Can you work these out from the model? Positions are in its coordinate system, mm. Coordinates: 2 decimals unless noted, no trailing zeros. Order: outer loops, then holes, each group sorted by start corner. A loop starts at its lowest first (then second) coordinate and runs counter-clockwise, first axis right, second up. Notation, with made-up numbers: (-15, 28.5) -> (40, 28.5) arc R24 cw to (40, 67.5) -> close; hole circle Ø2 at (73, 11.5). An arc over 180 degrees is marked (long way). Use a Markdown table: item, result. Add a question column.
1. Suppose I cut it at C-C, the plane z = 5.35. List the corners of the cut face in (x, y) for me, then the cut area to 3 significant figures.
2. Suppose I cut it at B-B, the plane x = -12.5. List the corners of the cut face in (y, z) for me, then the cut area to 3 significant figures.
3. Suppose I cut it at D-D, the plane z = 2.5. List the corners of the cut face in (x, y) for me, then the cut area to 3 significant figures.
4. We'd pull the mould along Y, two halves only. Please class faces 1 (the flat face through (-26, 41, 6.4)), 2 (the cylindrical face through (12.776, 26.96, 3.358)), 3 (the cylindrical face through (-17.594, -3.941, 2.372)): pulls with the +Y half, pulls with the -Y half, needs draft (parallel to the pull), parting line crosses it, or undercut.
5. Suppose I cut it at A-A, the plane y = 19. List the corners of the cut face in (x, z) for me, then the cut area to 3 significant figures.
6. If I drill on line 1 along Y through (x, z) = (-12.5, 1.7); line 2 along Y through (x, z) = (-21, 1.55); line 3 along X through (y, z) = (8, 0.7), over which ranges is the centre line in solid material (lowest first)? Write a range as from..to.
7. For pin 1 Ø1 at (x, z) = (2, 3.5) entering from -Y, with a flat end and sliding along its axis, tell me the tip position at first contact or that it passes through.
```python
from build123d import *

# Parameters (mm, degrees)
CYLINDER025_R     = 23.5
CYLINDER025_DEPTH = 6
CYLINDER024_R     = 26.5
CYLINDER024_DEPTH = 6
CHAMFER013_SIZE   = 2


with BuildPart() as obj1:
    # Cylinder025 → Cylinder025 (new body)
    with BuildSketch(Plane(origin=(-12.5, 19, -10.6), x_dir=(1, 0, 0), z_dir=(0, 0, 1))):
        Circle(CYLINDER025_R)
    extrude(amount=CYLINDER025_DEPTH)


with BuildPart() as obj2:
    # Cylinder024 → Cylinder024 (new body)
    with BuildSketch(Plane(origin=(-12.5, 19, -10.6), x_dir=(1, 0, 0), z_dir=(0, 0, 1))):
        Circle(CYLINDER024_R)
    extrude(amount=CYLINDER024_DEPTH)

    # Cut012: cut obj1
    add(obj1.part, mode=Mode.SUBTRACT)


with BuildPart() as obj2_1:
    # Cut012 placement: moved
    add(obj2.part.moved(Location((0, 0, 11))))

    # Chamfer013
    chamfer013_edges = [obj2_1.edges().sort_by_distance(p)[0] for p in [
        (-36, 19, 6.4),
    ]]
    chamfer(chamfer013_edges, length=CHAMFER013_SIZE)


solid = obj2_1.part
```
Worked out:
| question | item | result |
|---|---|---|
| 1 | outline | circle Ø53 at (-12.5, 19); hole circle Ø48.9 at (-12.5, 19) |
| 1 | area | 328 mm² |
| 2 | outline | (-7.5, 0.4) -> (-4.5, 0.4) -> (-4.5, 4.4) -> (-6.5, 6.4) -> (-7.5, 6.4) -> close; (42.5, 0.4) -> (45.5, 0.4) -> (45.5, 6.4) -> (44.5, 6.4) -> (42.5, 4.4) -> close |
| 2 | area | 32.0 mm² |
| 3 | outline | circle Ø53 at (-12.5, 19); hole circle Ø47 at (-12.5, 19) |
| 3 | area | 471 mm² |
| 4 | face 1 | needs draft |
| 4 | face 2 | parting line crosses it |
| 4 | face 3 | undercut |
| 5 | outline | (-39, 0.4) -> (-36, 0.4) -> (-36, 4.4) -> (-38, 6.4) -> (-39, 6.4) -> close; (11, 0.4) -> (14, 0.4) -> (14, 6.4) -> (13, 6.4) -> (11, 4.4) -> close |
| 5 | area | 32.0 mm² |
| 6 | line 1 | y = -7.5..-4.5, 42.5..45.5 |
| 6 | line 2 | y = -6.1..-2.91, 40.91..44.1 |
| 6 | line 3 | x = -36.61..-33.27, 8.27..11.61 |
| 7 | pin 1 | stops at y = -3.5 |
